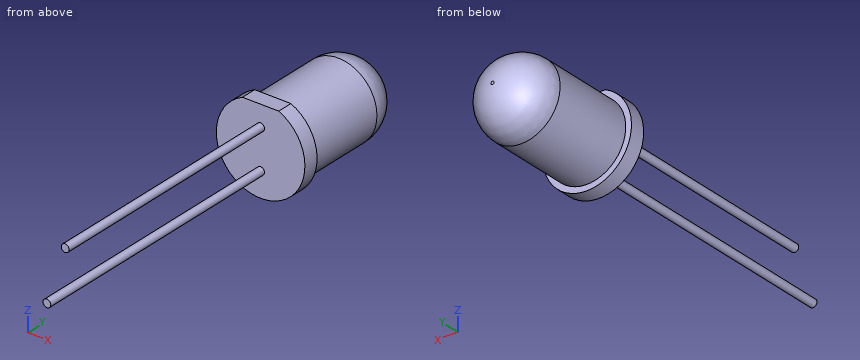
from build123d import *

# Parameters (mm, degrees)
CUT_EXTRUDE1_DEPTH  = 1
SKETCH3_R           = 0.25
BOSS_EXTRUDE1_DEPTH = 16
SKETCH4_R           = 0.25
BOSS_EXTRUDE2_DEPTH = 1.5


with BuildPart() as part:
    # Sketch1 → Revolve1 (revolve)
    with BuildSketch(Plane.XY):
        with BuildLine():
            Line((0, 0), (0, 8.75))
            Line((0, 8.75), (0.1, 8.75))
            ThreePointArc((0.1, 8.75), (1.782914139, 8.052914139), (2.48, 6.37))
            Line((2.48, 6.37), (2.48, 1))
            Line((2.48, 1), (2.85, 1))
            Line((2.85, 1), (2.85, 0))
            Line((2.85, 0), (0, 0))
        make_face()
    revolve(axis=Axis((0, 0, 0), (0, 1, 0)))

    # Sketch2 → Cut-Extrude1 (cut)
    with BuildSketch(Plane.XZ):
        with BuildLine():
            Line((-1.167261753, 2.6), (1.167261753, 2.6))
            ThreePointArc((1.167261753, 2.6), (0, 2.85), (-1.167261753, 2.6))
        make_face()
    extrude(amount=-CUT_EXTRUDE1_DEPTH, mode=Mode.SUBTRACT)

    # Sketch3 → Boss-Extrude1 (add)
    with BuildSketch(Plane.XZ):
        with Locations((0, -1.27)):
            Circle(SKETCH3_R)
        with Locations((0, 1.27)):
            Circle(SKETCH3_R)
    extrude(amount=BOSS_EXTRUDE1_DEPTH)

    # Sketch4 → Boss-Extrude2 (add)
    with BuildSketch(Plane.XZ.offset(16)):
        with Locations((0, -1.27)):
            Circle(SKETCH4_R)
    extrude(amount=BOSS_EXTRUDE2_DEPTH)


solid = part.part
Here's how the part is built. I have some questions about the finished solid (model axes, mm). Coordinates: 2 decimals unless noted, no trailing zeros. Order: outer loops, then holes, each group sorted by start corner. A loop starts at its lowest first (then second) coordinate and runs counter-clockwise, first axis right, second up.
Item 1: If we section it at B-B on y = 0.75: List the corners of the cut face in (x, z) for me.
Result sheet:
outline: (-1.17, 2.6) arc R2.85 ccw (long way) to (1.17, 2.6) - close
Item 2: For P1, Ø3, axis at y = -5.5, z = 1, coming from the -X side; P2, Ø1, axis at x = 0, y = -2.5, coming from the +Z side, each with a flat end and sliding along its axis, tell me the tip position at first contact or that it passes through.
Result sheet:
P1: stops at x = -0.25
P2: stops at z = 1.52
Item 3: I need wall thicknesses on line 1 (Z direction, x = 0.15, y = -10); line 2 (Y direction, x = 1.05, z = 2.4); line 3 (X direction, y = 6.5, z = -1.4). Which ranges of each line are inside material? Lowest first, please.
Result sheet:
line 1: z = -1.47 to -1.07, 1.07 to 1.47
line 2: y = 0 to 1
line 3: x = -2.04 to 2.04
Item 4: If we section it at A-A on y = -6.75: List the corners of the cut face in (x, z) for me.
Result sheet:
outline: circle Ø0.5 at (0, -1.27); circle Ø0.5 at (0, 1.27)
